```python
from build123d import *

# Parameters (mm, degrees)
SKETCH1_W           = 180
SKETCH1_H           = 75.87
BOSS_EXTRUDE1_DEPTH = 3


with BuildPart() as part:
    # Sketch1 → Boss-Extrude1 (new body)
    with BuildSketch(Plane(origin=(0, 0, 0), x_dir=(1, 0, 0), z_dir=(0, 1, 0))):
        with Locations((-5.566969943, 8.461475771)):
            Rectangle(SKETCH1_W, SKETCH1_H)
        with BuildLine():
            Line((-85.566969943, 25.396475771), (74.433030057, 25.396475771))
            ThreePointArc((74.433030057, 25.396475771), (75.433030057, 24.396475771), (74.433030057, 23.396475771))
            Line((74.433030057, 23.396475771), (-85.566969943, 23.396475771))
            ThreePointArc((-85.566969943, 23.396475771), (-86.566969943, 24.396475771), (-85.566969943, 25.396475771))
        make_face(mode=Mode.SUBTRACT)
        with BuildLine():
            Line((-85.566969943, 33.396475771), (74.433030057, 33.396475771))
            ThreePointArc((74.433030057, 33.396475771), (75.433030057, 32.396475771), (74.433030057, 31.396475771))
            Line((74.433030057, 31.396475771), (-85.566969943, 31.396475771))
            ThreePointArc((-85.566969943, 31.396475771), (-86.566969943, 32.396475771), (-85.566969943, 33.396475771))
        make_face(mode=Mode.SUBTRACT)
        with BuildLine():
            Line((-85.566969943, 17.396475771), (74.433030057, 17.396475771))
            ThreePointArc((74.433030057, 17.396475771), (75.433030057, 16.396475771), (74.433030057, 15.396475771))
            Line((74.433030057, 15.396475771), (-85.566969943, 15.396475771))
            ThreePointArc((-85.566969943, 15.396475771), (-86.566969943, 16.396475771), (-85.566969943, 17.396475771))
        make_face(mode=Mode.SUBTRACT)
        with BuildLine():
            Line((-85.566969943, 9.396475771), (74.433030057, 9.396475771))
            ThreePointArc((74.433030057, 9.396475771), (75.433030057, 8.396475771), (74.433030057, 7.396475771))
            Line((74.433030057, 7.396475771), (-85.566969943, 7.396475771))
            ThreePointArc((-85.566969943, 7.396475771), (-86.566969943, 8.396475771), (-85.566969943, 9.396475771))
        make_face(mode=Mode.SUBTRACT)
        with BuildLine():
            Line((-85.566969943, 1.396475771), (74.433030057, 1.396475771))
            ThreePointArc((74.433030057, 1.396475771), (75.433030057, 0.396475771), (74.433030057, -0.603524229))
            Line((74.433030057, -0.603524229), (-85.566969943, -0.603524229))
            ThreePointArc((-85.566969943, -0.603524229), (-86.566969943, 0.396475771), (-85.566969943, 1.396475771))
        make_face(mode=Mode.SUBTRACT)
        with BuildLine():
            Line((-85.566969943, -6.603524229), (74.433030057, -6.603524229))
            ThreePointArc((74.433030057, -6.603524229), (75.433030057, -7.603524229), (74.433030057, -8.603524229))
            Line((74.433030057, -8.603524229), (-85.566969943, -8.603524229))
            ThreePointArc((-85.566969943, -8.603524229), (-86.566969943, -7.603524229), (-85.566969943, -6.603524229))
        make_face(mode=Mode.SUBTRACT)
        with BuildLine():
            Line((-85.566969943, -14.603524229), (74.433030057, -14.603524229))
            ThreePointArc((74.433030057, -14.603524229), (75.433030057, -15.603524229), (74.433030057, -16.603524229))
            Line((74.433030057, -16.603524229), (-85.566969943, -16.603524229))
            ThreePointArc((-85.566969943, -16.603524229), (-86.566969943, -15.603524229), (-85.566969943, -14.603524229))
        make_face(mode=Mode.SUBTRACT)
    extrude(amount=BOSS_EXTRUDE1_DEPTH)


solid = part.part
```
Could you check a few things on this model? Use its own coordinates, in mm. A direction names the side the tool comes from. Round coordinates to 2 decimals unless told otherwise and drop trailing zeros. Write item = value, one per line.
1. I need wall thicknesses on probe 1 along X at (y, z) = (2.9, 15.5); probe 2 along X at (y, z) = (2.7, -15.5). Which ranges of each line are inside material? Lowest first, please.
Results below:
probe_1 = -95.57 to -86.56, 75.43 to 84.43
probe_2 = -95.57 to -86.01, 74.88 to 84.43
2. Which directions (+Z, -Z, +X, -X, +Y, -Y) give clear straight access to the entire face, cutting with the end or side of a thin tool? Please do faces 1 (the face through (84.433, 1, -8)), 2 (the face through (-4, 1, 16.604)).
Results below:
face_1 = +Z, -Z, +X, +Y, -Y
face_2 = +Y, -Y
3. I want a section at A-A, the plane x = 4.5. Count the separate pieces of the cut face and the enclosed holes in it, and give its area (3 significant figures).
Results below:
separate_pieces = 8
enclosed_holes = 0
area = 186 mm²
4. Thinking about a two-plate mould opening in Z: for faces 3 (the face through (-7, 1, -17.396)), 4 (the face through (-7, 1, -46.396)), 5 (the face through (-7, 0, -26)), which applies, +Z half, -Z half, draft (parallel to the pull), parting line (faces both ways), or undercut?
Results below:
face_3 = undercut
face_4 = -Z half
face_5 = draft
